```python
from build123d import *

# Parameters (mm, degrees)
SKETCH1_W           = 646.4808
SKETCH1_H           = 355.6
BOSS_EXTRUDE1_DEPTH = 5.4864
CUT_EXTRUDE1_DEPTH  = 738.847467539
CUT_EXTRUDE2_DEPTH  = 738.847467539


with BuildPart() as part:
    # Sketch1 → Boss-Extrude1 (new body)
    with BuildSketch(Plane.XY):
        with Locations((323.2404, 177.8)):
            Rectangle(SKETCH1_W, SKETCH1_H)
    extrude(amount=BOSS_EXTRUDE1_DEPTH)

    # Sketch4 → Cut-Extrude1 (cut, through all)
    with BuildSketch(Plane.XY.offset(5.4864)):
        with BuildLine():
            Line((424.8404, 177.8), (430.5808, 177.8))
            ThreePointArc((430.5808, 177.8), (432.4858, 175.895), (430.5808, 173.99))
            Line((430.5808, 173.99), (430.5808, 0))
            Line((430.5808, 0), (424.8404, 0))
            Line((424.8404, 0), (424.8404, 173.99))
            ThreePointArc((424.8404, 173.99), (422.9354, 175.895), (424.8404, 177.8))
        make_face()
        with BuildLine():
            Line((215.9, 177.8), (221.6404, 177.8))
            ThreePointArc((221.6404, 177.8), (223.5454, 175.895), (221.6404, 173.99))
            Line((221.6404, 173.99), (221.6404, 0))
            Line((221.6404, 0), (215.9, 0))
            Line((215.9, 0), (215.9, 173.99))
            ThreePointArc((215.9, 173.99), (213.995, 175.895), (215.9, 177.8))
        make_face()
    extrude(amount=-CUT_EXTRUDE1_DEPTH, mode=Mode.SUBTRACT)

    # Sketch5 → Cut-Extrude2 (cut, through all)
    with BuildSketch(Plane.XY.offset(5.4864)):
        with BuildLine():
            Line((0, 0), (12.7, 0))
            Line((12.7, 0), (12.7, 3.81))
            Line((12.7, 3.81), (12.7, 34.29))
            ThreePointArc((12.7, 34.29), (14.605, 36.195), (12.7, 38.1))
            Line((12.7, 38.1), (0, 38.1))
            ThreePointArc((0, 38.1), (-1.905, 36.195), (0, 34.29))
            Line((0, 34.29), (0, 3.81))
            ThreePointArc((0, 3.81), (-1.905, 1.905), (0, 0))
        make_face()
        with BuildLine():
            Line((0, 117.475), (12.7, 117.475))
            ThreePointArc((12.7, 117.475), (14.605, 115.57), (12.7, 113.665))
            Line((12.7, 113.665), (12.7, 83.185))
            ThreePointArc((12.7, 83.185), (14.605, 81.28), (12.7, 79.375))
            Line((12.7, 79.375), (0, 79.375))
            ThreePointArc((0, 79.375), (-1.905, 81.28), (0, 83.185))
            Line((0, 83.185), (0, 113.665))
            ThreePointArc((0, 113.665), (-1.905, 115.57), (0, 117.475))
        make_face()
        with BuildLine():
            Line((0, 196.85), (12.7, 196.85))
            ThreePointArc((12.7, 196.85), (14.605, 194.945), (12.7, 193.04))
            Line((12.7, 193.04), (12.7, 162.56))
            ThreePointArc((12.7, 162.56), (14.605, 160.655), (12.7, 158.75))
            Line((12.7, 158.75), (0, 158.75))
            ThreePointArc((0, 158.75), (-1.905, 160.655), (0, 162.56))
            Line((0, 162.56), (0, 193.04))
            ThreePointArc((0, 193.04), (-1.905, 194.945), (0, 196.85))
        make_face()
        with BuildLine():
            Line((0, 276.225), (12.7, 276.225))
            ThreePointArc((12.7, 276.225), (14.605, 274.32), (12.7, 272.415))
            Line((12.7, 272.415), (12.7, 241.935))
            ThreePointArc((12.7, 241.935), (14.605, 240.03), (12.7, 238.125))
            Line((12.7, 238.125), (0, 238.125))
            ThreePointArc((0, 238.125), (-1.905, 240.03), (0, 241.935))
            Line((0, 241.935), (0, 272.415))
            ThreePointArc((0, 272.415), (-1.905, 274.32), (0, 276.225))
        make_face()
        with BuildLine():
            Line((0, 355.6), (12.7, 355.6))
            Line((12.7, 355.6), (12.7, 351.79))
            Line((12.7, 351.79), (12.7, 321.31))
            ThreePointArc((12.7, 321.31), (14.605, 319.405), (12.7, 317.5))
            Line((12.7, 317.5), (0, 317.5))
            ThreePointArc((0, 317.5), (-1.905, 319.405), (0, 321.31))
            Line((0, 321.31), (0, 351.79))
            ThreePointArc((0, 351.79), (-1.905, 353.695), (0, 355.6))
        make_face()
        with BuildLine():
            Line((646.4808, 321.31), (646.4808, 351.79))
            ThreePointArc((646.4808, 351.79), (648.3858, 353.695), (646.4808, 355.6))
            Line((646.4808, 355.6), (633.7808, 355.6))
            Line((633.7808, 355.6), (633.7808, 351.79))
            Line((633.7808, 351.79), (633.7808, 321.31))
            ThreePointArc((633.7808, 321.31), (631.8758, 319.405), (633.7808, 317.5))
            Line((633.7808, 317.5), (646.4808, 317.5))
            ThreePointArc((646.4808, 317.5), (648.3858, 319.405), (646.4808, 321.31))
        make_face()
        with BuildLine():
            Line((646.4808, 241.935), (646.4808, 272.415))
            ThreePointArc((646.4808, 272.415), (648.3858, 274.32), (646.4808, 276.225))
            Line((646.4808, 276.225), (633.7808, 276.225))
            ThreePointArc((633.7808, 276.225), (631.8758, 274.32), (633.7808, 272.415))
            Line((633.7808, 272.415), (633.7808, 241.935))
            ThreePointArc((633.7808, 241.935), (631.8758, 240.03), (633.7808, 238.125))
            Line((633.7808, 238.125), (646.4808, 238.125))
            ThreePointArc((646.4808, 238.125), (648.3858, 240.03), (646.4808, 241.935))
        make_face()
        with BuildLine():
            Line((646.4808, 162.56), (646.4808, 193.04))
            ThreePointArc((646.4808, 193.04), (648.3858, 194.945), (646.4808, 196.85))
            Line((646.4808, 196.85), (633.7808, 196.85))
            ThreePointArc((633.7808, 196.85), (631.8758, 194.945), (633.7808, 193.04))
            Line((633.7808, 193.04), (633.7808, 162.56))
            ThreePointArc((633.7808, 162.56), (631.8758, 160.655), (633.7808, 158.75))
            Line((633.7808, 158.75), (646.4808, 158.75))
            ThreePointArc((646.4808, 158.75), (648.3858, 160.655), (646.4808, 162.56))
        make_face()
        with BuildLine():
            Line((646.4808, 83.185), (646.4808, 113.665))
            ThreePointArc((646.4808, 113.665), (648.3858, 115.57), (646.4808, 117.475))
            Line((646.4808, 117.475), (633.7808, 117.475))
            ThreePointArc((633.7808, 117.475), (631.8758, 115.57), (633.7808, 113.665))
            Line((633.7808, 113.665), (633.7808, 83.185))
            ThreePointArc((633.7808, 83.185), (631.8758, 81.28), (633.7808, 79.375))
            Line((633.7808, 79.375), (646.4808, 79.375))
            ThreePointArc((646.4808, 79.375), (648.3858, 81.28), (646.4808, 83.185))
        make_face()
        with BuildLine():
            Line((633.7808, 3.81), (633.7808, 34.29))
            ThreePointArc((633.7808, 34.29), (631.8758, 36.195), (633.7808, 38.1))
            Line((633.7808, 38.1), (646.4808, 38.1))
            ThreePointArc((646.4808, 38.1), (648.3858, 36.195), (646.4808, 34.29))
            Line((646.4808, 34.29), (646.4808, 3.81))
            ThreePointArc((646.4808, 3.81), (648.3858, 1.905), (646.4808, 0))
            Line((646.4808, 0), (633.7808, 0))
            Line((633.7808, 0), (633.7808, 3.81))
        make_face()
    extrude(amount=-CUT_EXTRUDE2_DEPTH, mode=Mode.SUBTRACT)


solid = part.part
```
Verification items for the finished model (mm, model axes). Round coordinates to 2 decimals unless told otherwise and drop trailing zeros. Loops run counter-clockwise (first coordinate to the right, second up) from the corner with the lowest first, then second, coordinate; pieces in that order, holes last. Notation, with made-up numbers: (10.25, 50) -> (40.25, 50) arc R12 ccw to (40.25, 66) -> close; hole circle Ø6 at (57.25, -34). An arc over 180 degrees is marked (long way). Answer as a JSON object with one key per item and string values.
Q1. Section check A-A (y = 149.5). Record the boundary of the cut face in (x, z).
Data:
{"outline": "(0, 0) -> (215.9, 0) -> (215.9, 5.49) -> (0, 5.49) -> close; (221.64, 0) -> (424.84, 0) -> (424.84, 5.49) -> (221.64, 5.49) -> close; (430.58, 0) -> (646.48, 0) -> (646.48, 5.49) -> (430.58, 5.49) -> close"}
Q2. Go/stop test with flat-tipped pins: P1, Ø1.6, axis at x = 643, z = 1.5, coming from the -Y side; P2, Ø1.6, axis at y = 177.5, z = 3, coming from the -X side; P3, Ø1.6, axis at y = 103.5, z = 1.5, coming from the +X side. Record where each tip stops, or that it passes through.
Data:
{"P1": "stops at y = 38.1", "P2": "stops at x = 12.7", "P3": "stops at x = 633.78"}
Q3. Scan lines: line 1 (X direction, y = 143, z = 5.1); line 2 (X direction, y = 88.5, z = 3.55); line 3 (Y direction, x = 431, z = 2.65). Record each from-to range of solid material in increasing order. Write a range as from..to.
Data:
{"line 1": "x = 0..215.9, 221.64..424.84, 430.58..646.48", "line 2": "x = 12.7..215.9, 221.64..424.84, 430.58..633.78", "line 3": "y = 0..174.04, 177.75..355.6"}
